from build123d import *

# Parameters (mm, degrees)
SKETCH1_W                   = 279.4
SKETCH1_H                   = 38.1
BOSS_EXTRUDE1_DEPTH         = 6.35
F_1_4_CLEARANCE_HOLE1_D     = 6.5278
F_1_4_CLEARANCE_HOLE1_DEPTH = 6.35


with BuildPart() as part:
    # Sketch1 → Boss-Extrude1 (new body)
    with BuildSketch(Plane(origin=(0, 0, 0), x_dir=(1, 0, 0), z_dir=(0, 1, 0))):
        Rectangle(SKETCH1_W, SKETCH1_H)
    extrude(amount=BOSS_EXTRUDE1_DEPTH)

    # 1/4 Clearance Hole1
    with Locations(Plane(origin=(0, 6.35, 0), x_dir=(-1, 0, 0), z_dir=(0, 1, 0))):
        with Locations((127, 12.7), (127, -12.7), (-127, -12.7), (-127, 12.7), (-88.9, -12.7), (-88.9, 12.7), (-50.8, -12.7), (-50.8, 12.7)):
            Hole(F_1_4_CLEARANCE_HOLE1_D / 2, depth=F_1_4_CLEARANCE_HOLE1_DEPTH)


solid = part.part
Could you check a few things on this model? Use its own coordinates, in mm. Give positions to 0.01 mm unless a question says otherwise; leave off trailing zeros. Order: outer loops, then holes, each group sorted by start corner. A loop starts at its lowest first (then second) coordinate and runs counter-clockwise, first axis right, second up.
Item 1: I need wall thicknesses on line 1 (Z direction, x = 88.9, y = 4); line 2 (X direction, y = 0.5, z = 15.5). Which ranges of each line are inside material? Lowest first, please.
Item 2: If we section it at C-C, the plane y = 2.25: Count the separate pieces of the cut face and the enclosed holes in it, plus the area to 3 significant figures.
Item 3: If we section it at B-B, the plane x = 88.9: Write out the boundary of the cut face in (y, z), plus the area to 3 significant figures.
Item 4: I'm going to push a flat-ended pin straight in: pin 1 (5 mm diameter, centred on x = 127, z = 12.7, fed in from -Y). Where does the tip first touch, or does it pass through?
Item 5: If we section it at A-A, the plane z = -12.7: Write out the boundary of the cut face in (x, y), plus the area to 3 significant figures.
Item 6: If we mould it in two halves opening along Z, with no side actions, what happens to faces 1 (the face through (-2, 3, -19.05)), 2 (the face through (123.74, 3.13, -12.56)), 3 (the face through (-2, 3, 19.05)), 4 (the face through (-2, 0, 0))? For each: pulls with the +Z half, pulls with the -Z half, needs draft (parallel to the pull), parting line crosses it, or undercut.
Values:
1. line 1: z = -19.05 to -15.96, -9.44 to 9.44, 15.96 to 19.05
1. line 2: x = -139.7 to -128.68, -125.32 to 49.12, 52.48 to 87.22, 90.58 to 125.32, 128.68 to 139.7
2. separate pieces: 1
2. enclosed holes: 8
2. area: 10,400 mm2
3. outline: (0, -19.05) - (6.35, -19.05) - (6.35, -15.96) - (0, -15.96) - close; (0, -9.44) - (6.35, -9.44) - (6.35, 9.44) - (0, 9.44) - close; (0, 15.96) - (6.35, 15.96) - (6.35, 19.05) - (0, 19.05) - close
3. area: 159 mm2
4. pin 1: passes through
5. outline: (-139.7, 0) - (-130.26, 0) - (-130.26, 6.35) - (-139.7, 6.35) - close; (-123.74, 0) - (47.54, 0) - (47.54, 6.35) - (-123.74, 6.35) - close; (54.06, 0) - (85.64, 0) - (85.64, 6.35) - (54.06, 6.35) - close; (92.16, 0) - (123.74, 0) - (123.74, 6.35) - (92.16, 6.35) - close; (130.26, 0) - (139.7, 0) - (139.7, 6.35) - (130.26, 6.35) - close
5. area: 1,610 mm2
6. face 1: pulls with the -Z half
6. face 2: undercut
6. face 3: pulls with the +Z half
6. face 4: needs draft
